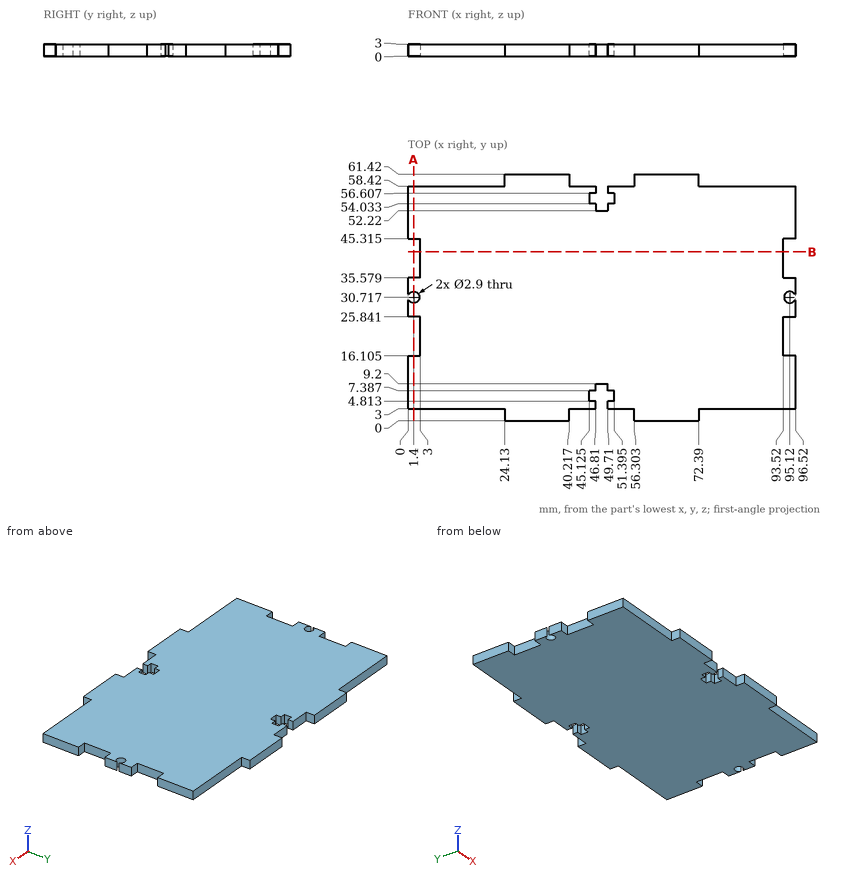
Answer from the drawing. Dimensions are ordinates in mm from the lowest x, y and z of the part. Give positions to 0.01 mm unless a question says otherwise; leave off trailing zeros. Write each loop counter-clockwise with the first axis right and the second up, starting at its lowest first coordinate (ties: lowest second). Pieces come first, ordered by that corner, then holes.
1) Find the intervals of material crossed by L1, parallel to Y at x = 1.4, z = 0.95 (1 decimal); L2, parallel to X at y = 57.5, z = 2.25; L3, parallel to Y at x = 91, z = 0.55, in increasing order.
2) Section A-A (x = 1.4) is taken. Write down the section's boundary in (y, z) (1 decimal).
3) Given P1, Ø1.5, axis at x = 82.5, z = 1.5, coming from the +Y side; P2, Ø1.5, axis at x = 49, z = 1, coming from the -Y side; P3, Ø0.9, axis at y = 38.5, z = 1, coming from the -X side, each flat-ended and moving along its own axis, determine where each tip first touches the part or whether it passes through.
4) Section B-B (y = 42) is taken. Write down the section's boundary in (x, z).
Response:
1. L1: y = 3 to 16.1, 25.8 to 29.3, 32.2 to 35.6, 45.3 to 58.4
1. L2: x = 0 to 46.81, 49.71 to 96.52
1. L3: y = 3 to 58.42
2. outline: (3, 0) - (16.1, 0) - (16.1, 3) - (3, 3) - close; (25.8, 0) - (29.3, 0) - (29.3, 3) - (25.8, 3) - close; (32.2, 0) - (35.6, 0) - (35.6, 3) - (32.2, 3) - close; (45.3, 0) - (58.4, 0) - (58.4, 3) - (45.3, 3) - close
3. P1: stops at y = 58.42
3. P2: stops at y = 3
3. P3: stops at x = 3
4. outline: (3, 0) - (93.52, 0) - (93.52, 3) - (3, 3) - close
